The model under review builds one solid part; all positions refer to its coordinate system, in mm. A direction names the side the tool comes from. Round coordinates to 2 decimals unless told otherwise and drop trailing zeros. Loops run counter-clockwise (first coordinate to the right, second up) from the corner with the lowest first, then second, coordinate; pieces in that order, holes last. Notation, with made-up numbers: M 40.25,-21.5 L 93.25,-21.5 A20 ccw 93.25,-9.5 Z; hole C 66,-11 d11. An arc over 180 degrees is marked long. One line per question, with ' | ' between items.
from build123d import *

# Parameters (mm, degrees)
F1_DEPTH = 4.826
F3_DEPTH = 25.4


with BuildPart() as f1:
    # F0 (on Top) → F1 (new body)
    with BuildSketch(Plane.XY):
        with BuildLine():
            Line((9.525, 0), (6.35, 0))
            ThreePointArc((6.35, 0), (4.4901280605, -4.4901280605), (0, -6.35))
            Line((0, -6.35), (5.4514567473, -7.810713433))
            ThreePointArc((5.4514567473, -7.810713433), (8.4454351729, -4.4045714594), (9.525, 0))
        make_face()
        with BuildLine():
            ThreePointArc((0, 6.35), (4.4901280605, 4.4901280605), (6.35, 0))
            Line((6.35, 0), (9.525, 0))
            ThreePointArc((9.525, 0), (8.4454351729, 4.4045714594), (5.4514567473, 7.810713433))
            Line((5.4514567473, 7.810713433), (0, 6.35))
        make_face()
        with BuildLine():
            Line((-5.4514567473, 7.810713433), (0, 6.35))
            Line((0, 6.35), (5.4514567473, 7.810713433))
            ThreePointArc((5.4514567473, 7.810713433), (0, 9.525), (-5.4514567473, 7.810713433))
        make_face()
        with BuildLine():
            ThreePointArc((-6.35, 0), (-4.4901280605, 4.4901280605), (0, 6.35))
            Line((0, 6.35), (-5.4514567473, 7.810713433))
            ThreePointArc((-5.4514567473, 7.810713433), (-8.4454351729, 4.4045714594), (-9.525, 0))
            Line((-9.525, 0), (-6.35, 0))
        make_face()
        with BuildLine():
            Line((-5.4514567473, -7.810713433), (0, -6.35))
            ThreePointArc((0, -6.35), (-4.4901280605, -4.4901280605), (-6.35, 0))
            Line((-6.35, 0), (-9.525, 0))
            ThreePointArc((-9.525, 0), (-8.4454351729, -4.4045714594), (-5.4514567473, -7.810713433))
        make_face()
        with BuildLine():
            Line((5.4514567473, -7.810713433), (0, -6.35))
            Line((0, -6.35), (-5.4514567473, -7.810713433))
            ThreePointArc((-5.4514567473, -7.810713433), (0, -9.525), (5.4514567473, -7.810713433))
        make_face()
        with BuildLine():
            Line((40.64, 0), (9.525, 0))
            ThreePointArc((9.525, 0), (8.4454351729, -4.4045714594), (5.4514567473, -7.810713433))
            Line((5.4514567473, -7.810713433), (34.3483223828, -15.5536052438))
            ThreePointArc((34.3483223828, -15.5536052438), (39.0075163, -8.3889785332), (40.64, 0))
        make_face()
        with BuildLine():
            ThreePointArc((5.4514567473, 7.810713433), (8.4454351729, 4.4045714594), (9.525, 0))
            Line((9.525, 0), (40.64, 0))
            ThreePointArc((40.64, 0), (39.0075163, 8.3889785332), (34.3483223828, 15.5536052438))
            Line((34.3483223828, 15.5536052438), (5.4514567473, 7.810713433))
        make_face()
        with BuildLine():
            ThreePointArc((-9.525, 0), (-8.4454351729, 4.4045714594), (-5.4514567473, 7.810713433))
            Line((-5.4514567473, 7.810713433), (-34.3483223828, 15.5536052438))
            ThreePointArc((-34.3483223828, 15.5536052438), (-39.0075163, 8.3889785332), (-40.64, 0))
            Line((-40.64, 0), (-9.525, 0))
        make_face()
        with BuildLine():
            Line((-34.3483223828, -15.5536052438), (-5.4514567473, -7.810713433))
            ThreePointArc((-5.4514567473, -7.810713433), (-8.4454351729, -4.4045714594), (-9.525, 0))
            Line((-9.525, 0), (-40.64, 0))
            ThreePointArc((-40.64, 0), (-39.0075163, -8.3889785332), (-34.3483223828, -15.5536052438))
        make_face()
    extrude(amount=F1_DEPTH)

    # F2 (on face) → F3 (cut)
    with BuildSketch(Plane.XY.offset(4.826)):
        with BuildLine():
            ThreePointArc((-33.5923079354, -7.4622272885), (-34.5892118857, -3.7901485539), (-34.925, 0))
            Line((-34.925, 0), (-37.1971782011, 0))
            ThreePointArc((-37.1971782011, 0), (-36.846066564, -4.0871759774), (-35.8030202404, -8.0545858653))
            Line((-35.8030202404, -8.0545858653), (-33.5923079354, -7.4622272885))
        make_face()
        with BuildLine():
            Line((-37.1971782011, 0), (-34.925, 0))
            ThreePointArc((-34.925, 0), (-33.5317746734, 7.6242904379), (-29.532176449, 14.2631228302))
            Line((-29.532176449, 14.2631228302), (-31.9856280478, 14.9205232048))
            ThreePointArc((-31.9856280478, 14.9205232048), (-35.8568057684, 7.9022507507), (-37.1971782011, 0))
        make_face()
        with BuildLine():
            Line((-31.9856280478, -14.9205232048), (-29.532176449, -14.2631228302))
            ThreePointArc((-29.532176449, -14.2631228302), (-30.8095695693, -12.6690899076), (-31.930357985, -10.9613113888))
            Line((-31.930357985, -10.9613113888), (-34.2169264562, -11.5739955641))
            ThreePointArc((-34.2169264562, -11.5739955641), (-33.1716116897, -13.294154894), (-31.9856280478, -14.9205232048))
        make_face()
        with BuildLine():
            ThreePointArc((-24.7160305152, -12.9726404166), (-28.0546836255, -6.8644949033), (-29.21, 0))
            Line((-29.21, 0), (-30.48, 0))
            ThreePointArc((-30.48, 0), (-29.3144832952, -7.0269524355), (-25.9427563146, -13.3013406039))
            Line((-25.9427563146, -13.3013406039), (-24.7160305152, -12.9726404166))
        make_face()
        with BuildLine():
            ThreePointArc((-26.2436859957, 10.7523729707), (-25.5155620849, 11.887072721), (-24.7160305152, 12.9726404166))
            Line((-24.7160305152, 12.9726404166), (-25.9427563146, 13.3013406039))
            ThreePointArc((-25.9427563146, 13.3013406039), (-26.731347274, 12.2119381475), (-27.4511523902, 11.075912616))
            Line((-27.4511523902, 11.075912616), (-26.2436859957, 10.7523729707))
        make_face()
        with BuildLine():
            Line((-30.48, 0), (-29.21, 0))
            ThreePointArc((-29.21, 0), (-28.8836587626, 3.6852190858), (-27.9147918493, 7.2557421873))
            Line((-27.9147918493, 7.2557421873), (-29.1181427694, 7.5781790945))
            ThreePointArc((-29.1181427694, 7.5781790945), (-30.1368303905, 3.8497874456), (-30.48, 0))
        make_face()
        with BuildLine():
            Line((-24.765, 0), (-23.495, 0))
            ThreePointArc((-23.495, 0), (-22.5758928334, 6.1114169896), (-19.8998845814, 11.6821580031))
            Line((-19.8998845814, 11.6821580031), (-21.1266103808, 12.0108581903))
            ThreePointArc((-21.1266103808, 12.0108581903), (-23.8354414226, 6.2749221806), (-24.765, 0))
        make_face()
        with BuildLine():
            ThreePointArc((-22.975438781, -4.6174457724), (-23.3647011405, -2.3232923472), (-23.495, 0))
            Line((-23.495, 0), (-24.765, 0))
            ThreePointArc((-24.765, 0), (-24.6214878009, -2.4883246732), (-24.192854341, -4.9436512885))
            Line((-24.192854341, -4.9436512885), (-22.975438781, -4.6174457724))
        make_face()
        with BuildLine():
            Line((-21.1266103808, -12.0108581903), (-19.8998845814, -11.6821580031))
            ThreePointArc((-19.8998845814, -11.6821580031), (-20.9260158473, -10.0078144461), (-21.789494801, -8.2440752881))
            Line((-21.789494801, -8.2440752881), (-22.9970709968, -8.5676443545))
            ThreePointArc((-22.9970709968, -8.5676443545), (-22.1399215448, -10.3316672167), (-21.1266103808, -12.0108581903))
        make_face()
        with BuildLine():
            ThreePointArc((-15.0837386475, -10.3916755895), (-17.09495644, -5.3678847519), (-17.78, 0))
            Line((-17.78, 0), (-19.05, 0))
            ThreePointArc((-19.05, 0), (-18.354285684, -5.5324386992), (-16.3104644469, -10.7203757767))
            Line((-16.3104644469, -10.7203757767), (-15.0837386475, -10.3916755895))
        make_face()
        with BuildLine():
            Line((-19.05, 0), (-17.78, 0))
            ThreePointArc((-17.78, 0), (-17.7211105613, 1.5855193171), (-17.544766757, 3.1623015892))
            Line((-17.544766757, 3.1623015892), (-18.7754484951, 3.4920617671))
            ThreePointArc((-18.7754484951, 3.4920617671), (-18.9812563815, 1.75141899), (-19.05, 0))
        make_face()
        with BuildLine():
            Line((-17.8611435758, 7.1914767497), (-16.6471026371, 6.8661754606))
            ThreePointArc((-16.6471026371, 6.8661754606), (-15.9451000092, 8.6642589099), (-15.0837386475, 10.3916755895))
            Line((-15.0837386475, 10.3916755895), (-16.3104644469, 10.7203757767))
            ThreePointArc((-16.3104644469, 10.7203757767), (-17.1620380999, 8.9894252693), (-17.8611435758, 7.1914767497))
        make_face()
        with BuildLine():
            Line((19.05, 0), (17.78, 0))
            ThreePointArc((17.78, 0), (17.09495644, -5.3678847519), (15.0837386475, -10.3916755895))
            Line((15.0837386475, -10.3916755895), (16.3104644469, -10.7203757767))
            ThreePointArc((16.3104644469, -10.7203757767), (18.354285684, -5.5324386992), (19.05, 0))
        make_face()
        with BuildLine():
            ThreePointArc((17.544766757, 3.1623015892), (17.7211105613, 1.5855193171), (17.78, 0))
            Line((17.78, 0), (19.05, 0))
            ThreePointArc((19.05, 0), (18.9812563815, 1.75141899), (18.7754484951, 3.4920617671))
            Line((18.7754484951, 3.4920617671), (17.544766757, 3.1623015892))
        make_face()
        with BuildLine():
            ThreePointArc((15.0837386475, 10.3916755895), (15.9451000092, 8.6642589099), (16.6471026371, 6.8661754606))
            Line((16.6471026371, 6.8661754606), (17.8611435758, 7.1914767497))
            ThreePointArc((17.8611435758, 7.1914767497), (17.1620380999, 8.9894252693), (16.3104644469, 10.7203757767))
            Line((16.3104644469, 10.7203757767), (15.0837386475, 10.3916755895))
        make_face()
        with BuildLine():
            ThreePointArc((19.8998845814, 11.6821580031), (22.5758928334, 6.1114169896), (23.495, 0))
            Line((23.495, 0), (24.765, 0))
            ThreePointArc((24.765, 0), (23.8354414226, 6.2749221806), (21.1266103808, 12.0108581903))
            Line((21.1266103808, 12.0108581903), (19.8998845814, 11.6821580031))
        make_face()
        with BuildLine():
            Line((24.765, 0), (23.495, 0))
            ThreePointArc((23.495, 0), (23.3647011405, -2.3232923472), (22.975438781, -4.6174457724))
            Line((22.975438781, -4.6174457724), (24.192854341, -4.9436512885))
            ThreePointArc((24.192854341, -4.9436512885), (24.6214878009, -2.4883246732), (24.765, 0))
        make_face()
        with BuildLine():
            ThreePointArc((21.789494801, -8.2440752881), (20.9260158473, -10.0078144461), (19.8998845814, -11.6821580031))
            Line((19.8998845814, -11.6821580031), (21.1266103808, -12.0108581903))
            ThreePointArc((21.1266103808, -12.0108581903), (22.1399215448, -10.3316672167), (22.9970709968, -8.5676443545))
            Line((22.9970709968, -8.5676443545), (21.789494801, -8.2440752881))
        make_face()
        with BuildLine():
            Line((30.48, 0), (29.21, 0))
            ThreePointArc((29.21, 0), (28.0546836255, -6.8644949033), (24.7160305152, -12.9726404166))
            Line((24.7160305152, -12.9726404166), (25.9427563146, -13.3013406039))
            ThreePointArc((25.9427563146, -13.3013406039), (29.3144832952, -7.0269524355), (30.48, 0))
        make_face()
        with BuildLine():
            ThreePointArc((27.9147918493, 7.2557421873), (28.8836587626, 3.6852190858), (29.21, 0))
            Line((29.21, 0), (30.48, 0))
            ThreePointArc((30.48, 0), (30.1368303905, 3.8497874456), (29.1181427694, 7.5781790945))
            Line((29.1181427694, 7.5781790945), (27.9147918493, 7.2557421873))
        make_face()
        with BuildLine():
            Line((25.9427563146, 13.3013406039), (24.7160305152, 12.9726404166))
            ThreePointArc((24.7160305152, 12.9726404166), (25.5155620849, 11.887072721), (26.2436859957, 10.7523729707))
            Line((26.2436859957, 10.7523729707), (27.4511523902, 11.075912616))
            ThreePointArc((27.4511523902, 11.075912616), (26.731347274, 12.2119381475), (25.9427563146, 13.3013406039))
        make_face()
        with BuildLine():
            ThreePointArc((29.532176449, 14.2631228302), (33.5317746734, 7.6242904379), (34.925, 0))
            Line((34.925, 0), (37.1971782011, 0))
            ThreePointArc((37.1971782011, 0), (35.8568057684, 7.9022507507), (31.9856280478, 14.9205232048))
            Line((31.9856280478, 14.9205232048), (29.532176449, 14.2631228302))
        make_face()
        with BuildLine():
            Line((37.1971782011, 0), (34.925, 0))
            ThreePointArc((34.925, 0), (34.5892118857, -3.7901485539), (33.5923079354, -7.4622272885))
            Line((33.5923079354, -7.4622272885), (35.8030202404, -8.0545858653))
            ThreePointArc((35.8030202404, -8.0545858653), (36.846066564, -4.0871759774), (37.1971782011, 0))
        make_face()
        with BuildLine():
            ThreePointArc((31.930357985, -10.9613113888), (30.8095695693, -12.6690899076), (29.532176449, -14.2631228302))
            Line((29.532176449, -14.2631228302), (31.9856280478, -14.9205232048))
            ThreePointArc((31.9856280478, -14.9205232048), (33.1716116897, -13.294154894), (34.2169264562, -11.5739955641))
            Line((34.2169264562, -11.5739955641), (31.930357985, -10.9613113888))
        make_face()
    extrude(amount=-F3_DEPTH, mode=Mode.SUBTRACT)


solid = f1.part
1) For line 1 (Y direction, x = -26.5, z = 2.8); line 2 (Y direction, x = 1, z = 2.55); line 3 (Y direction, x = -21.5, z = 2.25), list the stretches that pass through material, from the lowest coordinate up.
Output values:
line 1: y = -13.45 to -12.55, -10.31 to 10.82, 12.55 to 13.45 | line 2: y = -9.47 to -6.27, 6.27 to 9.47 | line 3: y = -12.11 to -11.43, -8.88 to 8.88, 11.43 to 12.11
2) Insertion check: P1, Ø2, axis at y = 7.5, z = 1, coming from the +X side; P2, Ø1, axis at x = -1, z = 3, coming from the +Y side; P3, Ø1, axis at x = 16, z = 2.5, coming from the -Y side. Each pin has a flat end and moves straight along its axis. Give the tip position at first contact, or say it passes through.
Output values:
P1: stops at x = 39.67 | P2: stops at y = 9.51 | P3: stops at y = -10.77
3) Add section B-B on y = -3.5. State how many separate pieces and enclosed holes the cut face has, then the cut area to 3 significant figures.
Output values:
separate pieces: 10 | enclosed holes: 0 | area: 279 mm²
4) Machinability: for faces 1 (the flat face through (10.2, -9.083, 2.379)), 2 (the flat face through (27.8, 13.8, 2.4)), 3 (the cylindrical face through (30.21, -3.43, 2.45)), which of the approach directions +Z, -Z, +X, -X, +Y, -Y give a long, thin tool a straight path to every point of the face, cutting with its end or side? Answer none if there is none.
Output values:
face 1: +Z, -Z, -Y | face 2: +Z, -Z, +Y | face 3: +Z, -Z
5) Add section A-A on x = -4. State the section outline as (y, z) points.
Output values:
outline: M -8.64,0 L -4.93,0 L -4.93,4.83 L -8.64,4.83 Z; M 4.93,0 L 8.64,0 L 8.64,4.83 L 4.93,4.83 Z
